Geometry: see drawing. Coordinates: mm, zero at the bounding-box minimum. A direction names the side the tool comes from. Coordinates: 2 decimals unless noted, no trailing zeros. Write each loop counter-clockwise with the first axis right and the second up, starting at its lowest first coordinate (ties: lowest second). Pieces come first, ordered by that corner, then holes.
1) Section query B-B (x = 22). Output: boundary loops of the cut face in (y, z).
2) Section query D-D (x = 6). Output: boundary loops of the cut face in (y, z).
3) Pin query (flat end, axial travel): pin 1 Ø11.5 at (x, z) = (22, 33) entering from -Y; pin 2 Ø13 at (x, z) = (29, 25.5) entering from -Y; pin 3 Ø6 at (x, y) = (35.5, 30.5) entering from -Z; pin 4 Ø1.5 at (x, y) = (28.5, 3.5) entering from +Z. Return the tip coordinate at first contact, or that it passes through.
4) Section query A-A (z = 33). Output: boundary loops of the cut face in (x, y), then the cut area to 3 significant figures.
5) Section query C-C (y = 8.5). Output: boundary loops of the cut face in (x, z).
6) Line query: L1, parallel to Z at x = 13.5, y = 3; L2, parallel to X at y = 16, z = 33; L3, parallel to X at y = 34, z = 33. Output: solid intervals per line, ascending.
7) Set-up query: the marked faces 1, 2, 3, 4 and 5. Return all of +Z, -Z, +X, -X, +Y, -Y with unobstructed straight access to the full face (end or side cutting, diameter ignored); none if empty.
8) Draft query along X for the marked faces 6, 7 and 8. Return one class per face: pulls with the +X half, pulls with the -X half, needs draft (parallel to the pull), parting line crosses it, or undercut.
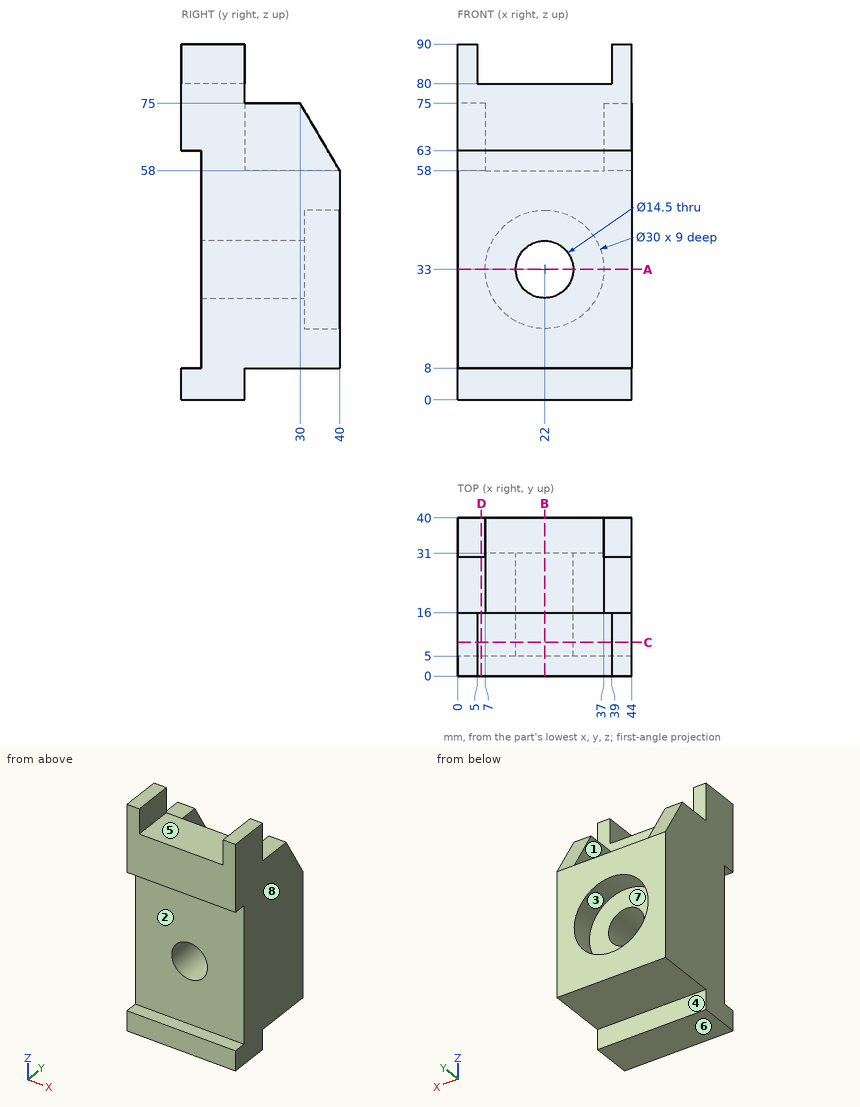
Answer:
1. outline: (0, 0) - (16, 0) - (16, 8) - (40, 8) - (40, 18) - (31, 18) - (31, 25.75) - (5, 25.75) - (5, 8) - (0, 8) - close; (0, 63) - (5, 63) - (5, 40.25) - (31, 40.25) - (31, 48) - (40, 48) - (40, 58) - (16, 58) - (16, 80) - (0, 80) - close
2. outline: (0, 0) - (16, 0) - (16, 8) - (40, 8) - (40, 58) - (30, 75) - (16, 75) - (16, 80) - (0, 80) - (0, 63) - (5, 63) - (5, 8) - (0, 8) - close
3. pin 1: passes through
3. pin 2: stops at y = 5
3. pin 3: stops at z = 8
3. pin 4: stops at z = 80
4. outline: (0, 5) - (14.75, 5) - (14.75, 31) - (7, 31) - (7, 40) - (0, 40) - close; (29.25, 5) - (44, 5) - (44, 40) - (37, 40) - (37, 31) - (29.25, 31) - close
4. area: 893 mm2
5. outline: (0, 0) - (44, 0) - (44, 90) - (39, 90) - (39, 80) - (5, 80) - (5, 90) - (0, 90) - close; hole circle Ø14.5 at (22, 33)
6. L1: z = 0 to 8, 63 to 80
6. L2: x = 0 to 14.75, 29.25 to 44
6. L3: x = 0 to 7, 37 to 44
7. face 1: +Z, +Y
7. face 2: +X, -X, -Y
7. face 3: +Y
7. face 4: -Z, +X, -X, +Y
7. face 5: +Z, +Y, -Y
8. face 6: needs draft
8. face 7: undercut
8. face 8: pulls with the +X half
